The figure shows three views and two pictorial views of one solid part (mm, origin at its lowest corner). Answer the questions. Give positions to 0.01 mm unless a question says otherwise; leave off trailing zeros. Order: outer loops, then holes, each group sorted by start corner. A loop starts at its lowest first (then second) coordinate and runs counter-clockwise, first axis right, second up. Notation, with made-up numbers: (71.5, -15.75) - (103.5, -15.75) arc R16 cw to (103.5, 10.25) - close; hole circle Ø4 at (87.25, 76). An arc over 180 degrees is marked (long way). Write item = value, one per line.
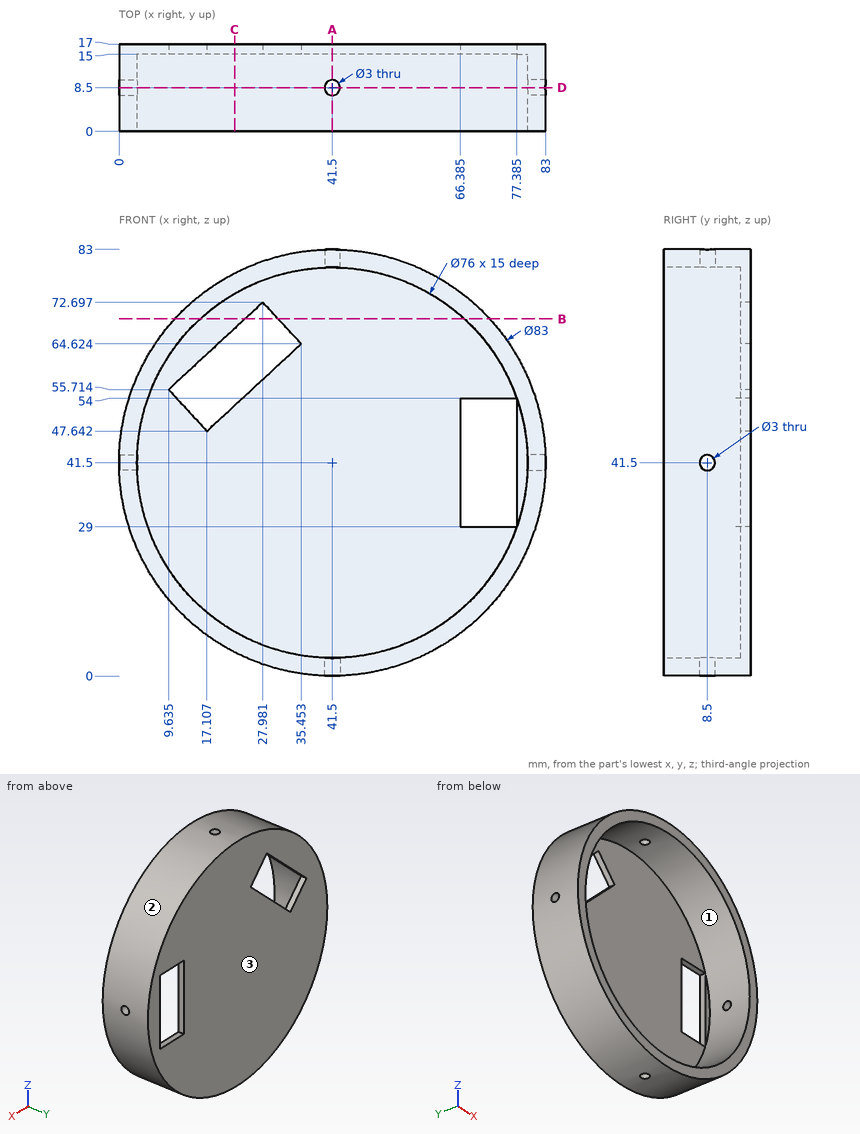
1. Determine the mould class of the marked faces 1, 2 and 3 for opening direction X: +X half, -X half, draft (parallel to the pull), parting line (faces both ways), or undercut.
Recorded:
face_1 = undercut
face_2 = parting line
face_3 = draft
2. Straight lines are drawn through the part: L1, parallel to Z at x = 41.5, y = 4.25; L2, parallel to Y at x = 15, z = 27.5; L3, parallel to Z at x = 24.5, y = 2.25 (1 decimal). For each, find the intervals that lie inside material, in ascending order. Write a range as [from, to].
Recorded:
L1 = [0, 3.5], [79.5, 83]
L2 = [15, 17]
L3 = [3.6, 7.5], [75.5, 79.4]
3. Section C-C (x = 22.5) is taken. Determine the outline of the cut face in (y, z) (1 decimal).
Recorded:
outline = (0, 4.6) - (17, 4.6) - (17, 52.6) - (15, 52.6) - (15, 8.6) - (0, 8.6) - close; (0, 74.4) - (15, 74.4) - (15, 67.6) - (17, 67.6) - (17, 78.4) - (0, 78.4) - close
4. Section D-D (y = 8.5) is taken. Determine the outline of the cut face in (x, z).
Recorded:
outline = (0.03, 40) arc R41.5 ccw to (40, 0.03) - (40, 3.53) arc R38 cw to (3.53, 40) - close; (0.03, 43) - (3.53, 43) arc R38 cw to (40, 79.47) - (40, 82.97) arc R41.5 ccw to start; (43, 0.03) arc R41.5 ccw to (82.97, 40) - (79.47, 40) arc R38 cw to (43, 3.53) - close; (43, 79.47) arc R38 cw to (79.47, 43) - (82.97, 43) arc R41.5 ccw to (43, 82.97) - close
5. Section B-B (z = 69.5) is taken. Determine the outline of the cut face in (x, y).
Recorded:
outline = (10.87, 0) - (15.81, 0) - (15.81, 15) - (24.53, 15) - (24.53, 17) - (10.87, 17) - close; (30.94, 15) - (67.19, 15) - (67.19, 0) - (72.13, 0) - (72.13, 17) - (30.94, 17) - close
6. Flat-ended cylindrical pins translate along their axes: pin 1 (0.6 mm diameter, centred on x = 73.5, y = 15.5, fed in from +Z) (1 decimal); pin 2 (0.6 mm diameter, centred on y = 15.5, z = 47.5, fed in from -X); pin 3 (8 mm diameter, centred on x = 46, y = 2, fed in from +Z). Find the tip coordinate at first contact, or state that the pin passes through.
Recorded:
pin_1 = 68.3
pin_2 = 0.39
pin_3 = 83
7. Section A-A (x = 41.5) is taken. Determine the outline of the cut face in (y, z).
Recorded:
outline = (0, 0) - (7, 0) - (7, 3.5) - (0, 3.5) - close; (0, 79.5) - (7, 79.5) - (7, 83) - (0, 83) - close; (10, 0) - (17, 0) - (17, 83) - (10, 83) - (10, 79.5) - (15, 79.5) - (15, 3.5) - (10, 3.5) - close
